Work out the finished part from the listing and answer in its coordinate system (mm). A direction names the side the tool comes from. Round coordinates to 2 decimals unless told otherwise and drop trailing zeros. Order: outer loops, then holes, each group sorted by start corner. A loop starts at its lowest first (then second) coordinate and runs counter-clockwise, first axis right, second up. Notation, with made-up numbers: (-6, 16) -> (2, 16) arc R21 cw to (2, 35) -> close; hole circle Ø2 at (28, 79). An arc over 180 degrees is marked (long way). Use one line per item in the form item = value.
```python
from build123d import *

# Parameters (mm, degrees)
BOSS_EXTRUDE1_DEPTH = 1.8
FILLET1_R           = 0.5
SKETCH5_R           = 2.5
SKETCH5_R_2         = 1.75
BOSS_EXTRUDE2_DEPTH = 1.8
FILLET2_R           = 1
CUT_EXTRUDE1_DEPTH  = 86.48993183
FILLET3_R           = 0.5


with BuildPart() as part:
    # Sketch1 → Boss-Extrude1 (new body)
    with BuildSketch(Plane.XY):
        with BuildLine():
            Line((0, 4.5), (0, 6.5))
            Line((0, 6.5), (6.1, 6.5))
            Line((6.1, 6.5), (6.1, 10.5))
            Line((6.1, 10.5), (10, 14.4))
            Line((10, 14.4), (10, 83.5))
            Line((10, 83.5), (16.4, 83.5))
            ThreePointArc((16.4, 83.5), (17.745328581, 80.945017946), (18.212299295, 78.095495067))
            Line((18.212299295, 78.095495067), (18.25, 49.5))
            Line((18.25, 49.5), (12, 49.5))
            Line((12, 49.5), (12, 37.18))
            add(Edge.make_bspline(
                [(12, 37.18), (12, 35.554764974), (12.5, 33.972282338), (12.5, 32.33)],
                knots=[0, 0, 0, 0, 1, 1, 1, 1], degree=3))
            Line((12.5, 32.33), (12.5, 3.07))
            ThreePointArc((12.5, 3.07), (11.600817818, 0.899182182), (9.43, 0))
            ThreePointArc((9.43, 0), (4.205660329, 1.182650422), (0, 4.5))
        make_face()
    extrude(amount=BOSS_EXTRUDE1_DEPTH)

    # Fillet1
    fillet1_edges = [part.edges().sort_by_distance(p)[0] for p in [
        (0, 6.5, 0.9),
        (6.1, 6.5, 0.9),
        (6.1, 10.5, 0.9),
        (10, 14.4, 0.9),
        (10, 83.5, 0.9),
        (18.25, 49.5, 0.9),
        (12, 49.5, 0.9),
    ]]
    fillet(fillet1_edges, radius=FILLET1_R)

    # Sketch5 → Boss-Extrude2 (add)
    # profile 1 of 3: a face of its own
    with BuildSketch(Plane(origin=(0, 0, 0), x_dir=(-1, 0, 0), z_dir=(0, 0, -1))):
        with Locations((-9.5, -2.499832541)):
            Circle(SKETCH5_R)
        with Locations((-9.5, -2.499832541)):
            Circle(SKETCH5_R_2, mode=Mode.SUBTRACT)
    # profile 2 of 3: a face of its own
    with BuildSketch(Plane(origin=(0, 0, 0), x_dir=(-1, 0, 0), z_dir=(0, 0, -1))):
        with BuildLine():
            ThreePointArc((-11.824045318, -1.578521867), (-9.031018815, -0.044215175), (-7, -2.499832541))
            Line((-7, -2.499832541), (-7, 0.245881701))
            ThreePointArc((-7, 0.245881701), (-8.2087959, 0.061626967), (-9.43, 0))
            ThreePointArc((-9.43, 0), (-10.256451345, 0.113333266), (-11.021883517, 0.444965358))
            Line((-11.021883517, 0.444965358), (-11.824045318, -1.578521867))
        make_face()
    # profile 3 of 3: a face of its own
    with BuildSketch(Plane(origin=(0, 0, 0), x_dir=(-1, 0, 0), z_dir=(0, 0, -1))):
        with BuildLine():
            ThreePointArc((-9.43, 0), (-8.2087959, 0.061626967), (-7, 0.245881701))
            Line((-7, 0.245881701), (-7, 0.500167459))
            Line((-7, 0.500167459), (-11, 0.500167459))
            Line((-11, 0.500167459), (-11.021883517, 0.444965358))
            ThreePointArc((-11.021883517, 0.444965358), (-10.256451345, 0.113333266), (-9.43, 0))
        make_face()
    extrude(amount=-BOSS_EXTRUDE2_DEPTH)

    # Fillet2
    fillet2_edges = [part.edges().sort_by_distance(p)[0] for p in [
        (7, 0.245881701, 0.9),
        (11.021883517, 0.444965358, 0.9),
    ]]
    fillet(fillet2_edges, radius=FILLET2_R)

    # Sketch6 → Cut-Extrude1 (cut, through all)
    with BuildSketch(Plane.XY.offset(1.8)):
        Polygon((10, 23.170696855), (10, 3.27), (15.071898879, 3.27), (15.071898879, -7.898815654), (-3.496989456, -7.898815654), (-3.496989456, 23.170696855), align=None)
    extrude(amount=-CUT_EXTRUDE1_DEPTH, mode=Mode.SUBTRACT)

    # Fillet3
    fillet3_edges = [part.edges().sort_by_distance(p)[0] for p in [
        (12.5, 3.27, 0.9),
        (10, 3.27, 0.9),
    ]]
    fillet(fillet3_edges, radius=FILLET3_R)


solid = part.part
```
Item 1: The part is cut by section B-B, the plane x = 15.25. Give the vertices of the cut face in (y, z).
Findings:
outline = (49.5, 0) -> (83.5, 0) -> (83.5, 1.8) -> (49.5, 1.8) -> close
Item 2: The part is cut by section A-A, the plane y = 19.5. Give the vertices of the cut face in (x, z).
Findings:
outline = (10, 0) -> (12.5, 0) -> (12.5, 1.8) -> (10, 1.8) -> close
Item 3: Consider line 1 along Y through (x, z) = (14.5, 1.5); line 2 along X through (y, z) = (70.5, 0.55); line 3 along X through (y, z) = (31, 0.1). Determine where each line is inside the solid, lowest interval first.
Findings:
line_1 = 49.5 to 83.5
line_2 = 10 to 18.22
line_3 = 10 to 12.5
Item 4: A flat-ended cylindrical pin translates along its axis: P1, Ø1, axis at y = 30, z = 0, coming from the +X side. Find the tip coordinate at first contact, or state that the pin passes through.
Findings:
P1 = 12.5
Item 5: For faces 1 (the flat face through (10, 43, 1)), 2 (the flat face through (12, 43, 1)), 3 (the flat face through (12.5, 18, 1)), determine the directions among +Z, -Z, +X, -X, +Y, -Y from which every point of the face is accessible in a straight line to the end or side of a thin tool.
Findings:
face_1 = +Z, -Z, -X, +Y, -Y
face_2 = +Z, -Z, +X
face_3 = +Z, -Z, +X, -Y
